```python
from build123d import *

# Parameters (mm, degrees)
SKETCH_W            = 116.082786
SKETCH_H            = 47.133754
PAD_DEPTH           = 4
SKETCH001_W         = 104.335838
SKETCH001_H         = 3.503182
POCKET_DEPTH        = 9
LINEARPATTERN_COUNT = 6
LINEARPATTERN_PITCH = 7.6
SKETCH002_W         = 4.652203
SKETCH002_H         = 4.844048
SKETCH003_W         = 4.652203
SKETCH003_H         = 4.844048
SKETCH004_W         = 4.84
SKETCH004_H         = 4.84
SKETCH005_W         = 4.84
SKETCH005_H         = 4.84
SKETCH006_W         = 4.84
SKETCH006_H         = 4.84
SKETCH007_W         = 4.84
SKETCH007_H         = 4.84
SKETCH008_W         = 4.84
SKETCH008_H         = 4.84
SKETCH009_W         = 4.84
SKETCH009_H         = 4.84


with BuildPart() as part:
    # Sketch → Pad (new body)
    with BuildSketch(Plane.XY):
        Rectangle(SKETCH_W, SKETCH_H)
    extrude(amount=PAD_DEPTH)

    # Sketch001 (on Face6 of Pad) → Pocket (cut)
    with BuildSketch(Plane.XY.offset(4)):
        with Locations((0, 18.245884)):
            Rectangle(SKETCH001_W, SKETCH001_H)
    pocket = extrude(amount=-POCKET_DEPTH, mode=Mode.SUBTRACT)

    # LinearPattern: Pocket ×6
    with Locations(*[(0, -i * LINEARPATTERN_PITCH, 0) for i in range(1, LINEARPATTERN_COUNT)]):
        add(pocket, mode=Mode.SUBTRACT)

    # Sketch002 (on Face4 of LinearPattern) → AdditiveLoft section 0
    with BuildSketch(Plane(origin=(0, 0, 0), x_dir=(1, 0, 0), z_dir=(0, 0, -1))):
        with Locations((-55.65727, 21.038372)):
            Rectangle(SKETCH002_W, SKETCH002_H)
    # Sketch003 (on Face4 of LinearPattern) → AdditiveLoft section 1
    with BuildSketch(Plane(origin=(-10, -10, -50), x_dir=(1, 0, 0), z_dir=(0, 0, -1))):
        with Locations((-55.65727, 21.038372)):
            Rectangle(SKETCH003_W, SKETCH003_H)
    loft()

    # Sketch004 (on Face4 of AdditiveLoft) → AdditiveLoft001 section 0
    with BuildSketch(Plane(origin=(0, 0, 0), x_dir=(1, 0, 0), z_dir=(0, 0, -1))):
        with Locations((55.627524, 21.025991)):
            Rectangle(SKETCH004_W, SKETCH004_H)
    # Sketch005 (on Face4 of AdditiveLoft) → AdditiveLoft001 section 1
    with BuildSketch(Plane(origin=(10, -10, -50), x_dir=(1, 0, 0), z_dir=(0, 0, -1))):
        with Locations((55.627524, 21.025991)):
            Rectangle(SKETCH005_W, SKETCH005_H)
    loft()

    # Sketch006 (on Face4 of AdditiveLoft001) → AdditiveLoft002 section 0
    with BuildSketch(Plane(origin=(0, 0, 0), x_dir=(1, 0, 0), z_dir=(0, 0, -1))):
        with Locations((-55.457449, -21.029405)):
            Rectangle(SKETCH006_W, SKETCH006_H)
    # Sketch007 (on Face4 of AdditiveLoft001) → AdditiveLoft002 section 1
    with BuildSketch(Plane(origin=(-10, 10, -50), x_dir=(1, 0, 0), z_dir=(0, 0, -1))):
        with Locations((-55.457449, -21.029405)):
            Rectangle(SKETCH007_W, SKETCH007_H)
    loft()

    # Sketch008 (on Face4 of AdditiveLoft002) → AdditiveLoft003 section 0
    with BuildSketch(Plane(origin=(0, 0, 0), x_dir=(1, 0, 0), z_dir=(0, 0, -1))):
        with Locations((55.563696, -21.007741)):
            Rectangle(SKETCH008_W, SKETCH008_H)
    # Sketch009 (on Face4 of AdditiveLoft002) → AdditiveLoft003 section 1
    with BuildSketch(Plane(origin=(10, 10, -50), x_dir=(1, 0, 0), z_dir=(0, 0, -1))):
        with Locations((55.563696, -21.007741)):
            Rectangle(SKETCH009_W, SKETCH009_H)
    loft()


solid = part.part
```
For this review, take the finished solid that the model builds, in its own axes (mm). A direction names the side the tool comes from. Give positions to 0.01 mm unless a question says otherwise; leave off trailing zeros. Write each loop counter-clockwise with the first axis right and the second up, starting at its lowest first coordinate (ties: lowest second). Pieces come first, ordered by that corner, then holes.
Item 1: Take a section at B-B (z = -22). Give the number of separate pieces and of enclosed holes in the cut face, and give its area (3 significant figures).
Item 2: The part is to be moulded in two halves that separate along Y. For faces 1 (the face through (-58.041, 0, 2)), 2 (the face through (-52.168, 18, 2)), say which applies: +Y half, -Y half, draft (parallel to the pull), parting line (faces both ways), or undercut.
Item 3: Take a section at A-A (x = -33). Give the boundary of the cut face in (y, z), and give its area (3 significant figures).
Item 4: Machinability: for faces 3 (the face through (52.168, 3, 2)), 4 (the face through (65, 31, -50)), which of the approach directions +Z, -Z, +X, -X, +Y, -Y give a long, thin tool a straight path to every point of the face, cutting with its end or side? Answer none if there is none.
Item 5: Wall thickness on probe 1 along Z at (x, y) = (2, -15.5): over which ranges is the line inside the solid? List them lowest first.
Item 6: Insertion check: P1, Ø3, axis at x = 44, y = -5.5, coming from the +Z side; P2, Ø12, axis at y = 6, z = -3, coming from the -X side; P3, Ø1.2, axis at x = -2, z = 1.5, coming from the -Y side; P4, Ø5, axis at y = -20.5, z = -31, coming from the -X side. Each pin has a flat end and moves straight along its axis. Give the tip position at first contact, or say it passes through.
Established:
1. separate pieces: 4
1. enclosed holes: 0
1. area: 92.8 mm2
2. face 1: draft
2. face 2: undercut
3. outline: (-23.57, 0) - (-21.51, 0) - (-21.51, 4) - (-23.57, 4) - close; (-18, 0) - (-13.91, 0) - (-13.91, 4) - (-18, 4) - close; (-10.4, 0) - (-6.31, 0) - (-6.31, 4) - (-10.4, 4) - close; (-2.8, 0) - (1.29, 0) - (1.29, 4) - (-2.8, 4) - close; (4.8, 0) - (8.89, 0) - (8.89, 4) - (4.8, 4) - close; (12.4, 0) - (16.49, 0) - (16.49, 4) - (12.4, 4) - close; (20, 0) - (23.57, 0) - (23.57, 4) - (20, 4) - close
3. area: 104 mm2
4. face 3: +Z, -Z
4. face 4: -Z, +X, -X, +Y, -Y
5. probe 1: z = 0 to 4
6. P1: stops at z = 4
6. P2: stops at x = -58.04
6. P3: stops at y = -23.57
6. P4: passes through
